from build123d import *

# Parameters (mm, degrees)
SKETCH2_W           = 30
SKETCH2_H           = 30
BOSS_EXTRUDE1_DEPTH = 50
SKETCH3_W           = 25
SKETCH3_H           = 25
CUT_EXTRUDE1_DEPTH  = 2.5
FILLET1_R           = 5
CUT_EXTRUDE2_DEPTH  = 61.207972969


with BuildPart() as part:
    # Sketch2 → Boss-Extrude1 (new body)
    with BuildSketch(Plane(origin=(0, 0, 0), x_dir=(1, 0, 0), z_dir=(0, 1, 0))):
        Rectangle(SKETCH2_W, SKETCH2_H)
    extrude(amount=BOSS_EXTRUDE1_DEPTH)

    # Sketch3 → Cut-Extrude1 (cut)
    with BuildSketch(Plane(origin=(0, 50, 0), x_dir=(1, 0, 0), z_dir=(0, 1, 0))):
        Rectangle(SKETCH3_W, SKETCH3_H)
    extrude(amount=-CUT_EXTRUDE1_DEPTH, mode=Mode.SUBTRACT)

    # Fillet1
    fillet1_edges = [part.edges().sort_by_distance(p)[0] for p in [
        (15, 25, 15),
        (-15, 25, 15),
        (-15, 25, -15),
        (15, 25, -15),
    ]]
    fillet(fillet1_edges, radius=FILLET1_R)

    # Cut-Loft2: read off the stored shape, not the designer's step
    # Cut-Loft2: loft between two sections, ruled curve by curve
    cut_loft2_from = [
        Edge.make_bspline([(0, 0, -12.5), (-25, 0, -12.5), (-25, 0, 12.5), (0, 0, 12.5), (25, 0, 12.5), (25, 0, -12.5), (0, 0, -12.5)], [0, 0, 0, 0, 0.5, 0.5, 0.5, 1, 1, 1, 1], 3, [1, 0.333333333, 0.333333333, 1, 0.333333333, 0.333333333, 1]),
    ]
    cut_loft2_to = [
        Edge.make_bspline([(0.784484005, 47.5, -2.373728048), (-3.962972092, 47.5, -3.942696057), (-5.531940101, 47.5, 0.804760039), (-0.784484005, 47.5, 2.373728048), (3.962972092, 47.5, 3.942696057), (5.531940101, 47.5, -0.804760039), (0.784484005, 47.5, -2.373728048)], [0, 0, 0, 0, 0.5, 0.5, 0.5, 1, 1, 1, 1], 3, [1, 0.333333333, 0.333333333, 1, 0.333333333, 0.333333333, 1]),
    ]
    cut_loft2 = Solid(Shell([*[Face.make_surface_from_curves(cut_loft2_from[k], cut_loft2_to[k]) for k in range(1)], Face(Wire(cut_loft2_from)), Face(Wire(cut_loft2_to))]))
    add(cut_loft2, mode=Mode.SUBTRACT)

    # Sketch9 → Cut-Extrude2 (cut, through all)
    with BuildSketch(Plane.XY.offset(15)):
        with BuildLine():
            Line((15, 50), (10, 50))
            Line((10, 50), (10, 46.180339887))
            ThreePointArc((10, 46.180339887), (13.693063938, 41.123724357), (15, 35))
            Line((15, 35), (15, 50))
        make_face()
        with BuildLine():
            Line((10, 50), (0, 50))
            ThreePointArc((0, 50), (5.352331347, 49.012585384), (10, 46.180339887))
            Line((10, 46.180339887), (10, 50))
        make_face()
    extrude(amount=-CUT_EXTRUDE2_DEPTH, mode=Mode.SUBTRACT)


solid = part.part
Can you work these out from the model? Positions are in its coordinate system, mm. A direction names the side the tool comes from. Coordinates: 2 decimals unless noted, no trailing zeros. Answer as a JSON object with one key per item and string values. Group by question number.
Item 1: For pin 1 (1 mm diameter, centred on x = -9, z = -10, fed in from +Y), with a flat end and sliding along its axis, tell me the tip position at first contact or that it passes through.
Item 2: If I drill on L1, parallel to Y at x = 7, z = -11.5; L2, parallel to X at y = 5, z = 2.5; L3, parallel to X at y = 20, z = 3, over which ranges is the centre line in solid material (lowest first)? Write a range as from..to.
Item 3: If we mould it in two halves opening along Z, with no side actions, what happens to faces 3 (the face through (-14, 25, -13)), 4 (the face through (-2, 49, 12.5)), 5 (the face through (0, 25, 15))? For each: released by +Z, released by -Z, zero draft, split by the parting line, or undercut.
Item 4: On a 3-axis mill with a long thin cutter (end or side, diameter ignored), from which of +Z, -Z, +X, -X, +Y, -Y can I reach the whole of each face in a straight line? I mean faces 1 (the face through (-12.5, 49, 0)), 2 (the face through (-15, 25, 0)). Say none if no direction works.
Returned:
{
 "1": {"pin 1": "stops at y = 47.5"},
 "2": {"L1": "y = 0..47.5", "L2": "x = -15..-11.16, 11.16..15", "L3": "x = -15..-7.68, 7.68..15"},
 "3": {"face 3": "released by -Z", "face 4": "undercut", "face 5": "released by +Z"},
 "4": {"face 1": "+X, +Y", "face 2": "+Z, -Z, -X, +Y, -Y"}
}
